```python
from build123d import *

# Parameters (mm, degrees)
SKETCH1_R           = 4
BOSS_EXTRUDE1_DEPTH = 8
CHAMFER1_SIZE       = 0.25
CUT_EXTRUDE1_DEPTH  = 3
CHAMFER2_SIZE       = 0.25


with BuildPart() as part:
    # Sketch1 → Boss-Extrude1 (new body)
    with BuildSketch(Plane(origin=(0, 0, 0), x_dir=(1, 0, 0), z_dir=(0, 1, 0))):
        with Locations(Location((0, 0, 0), (0, 0, 270))):
            Circle(SKETCH1_R)
    extrude(amount=-BOSS_EXTRUDE1_DEPTH)

    # Chamfer1
    chamfer1_edges = [part.edges().sort_by_distance(p)[0] for p in [
        (0, 0, -4),
        (0, -8, -4),
    ]]
    chamfer(chamfer1_edges, length=CHAMFER1_SIZE)

    # Sketch2 → Cut-Extrude1 (cut)
    with BuildSketch(Plane(origin=(0, 0, 0), x_dir=(1, 0, 0), z_dir=(0, 1, 0))):
        Polygon((0, 2.309401077), (2, 1.154700538), (2, -1.154700538), (0, -2.309401077), (-2, -1.154700538), (-2, 1.154700538), align=None)
    extrude(amount=-CUT_EXTRUDE1_DEPTH, mode=Mode.SUBTRACT)

    # Chamfer2
    chamfer2_edges = [part.edges().sort_by_distance(p)[0] for p in [
        (-1, 0, -1.732050808),
        (-2, 0, 0),
        (-1, 0, 1.732050808),
        (1, 0, 1.732050808),
        (2, 0, 0),
        (1, 0, -1.732050808),
    ]]
    chamfer(chamfer2_edges, length=CHAMFER2_SIZE)


solid = part.part
```
Geometry: final body of the model. Coordinates: model frame, mm. A direction names the side the tool comes from. Give positions to 0.01 mm unless a question says otherwise; leave off trailing zeros. Write each loop counter-clockwise with the first axis right and the second up, starting at its lowest first coordinate (ties: lowest second). Pieces come first, ordered by that corner, then holes.
1. Section query C-C, the plane y = -3.5. Return loops of the section in (x, z), then the cut area to 3 significant figures.
2. Section query B-B, the plane z = 0. Return loops of the section in (x, y).
3. Pin query (flat end, axial travel): P1, Ø4, axis at x = -1.5, y = -2, coming from the -Z side; P2, Ø1.5, axis at x = 2.5, y = -3.5, coming from the +Z side; P3, Ø1, axis at y = -5, z = -1, coming from the -X side. Return the tip coordinate at first contact, or that it passes through.
4. Section query A-A, the plane y = -1.5. Return loops of the section in (x, z).
5. Line query: probe 1 along X at (y, z) = (-0.75, -2); probe 2 along Z at (x, y) = (-1.5, -2.5); probe 3 along Z at (x, y) = (3, -2.25). Output: solid intervals per line, ascending.
6. Draft query along Z for faces 1 (the flat face through (1.046, -0.127, -1.848)), 2 (the flat face through (0, -8, 0)), 3 (the cylindrical face through (-3.905, -3.948, -0.867)). Return one class per face: released by +Z, released by -Z, zero draft, split by the parting line, or undercut.
7. Reachability of faces 4 (the flat face through (-2, -2, 0)), 5 (the flat face through (2, 0, 2)) from +Z, -Z, +X, -X, +Y, -Y: full face, straight path, thin tool, end or side. Return the list, or none.
Computed:
1. outline: circle Ø8 at (0, 0)
1. area: 50.3 mm2
2. outline: (-4, -7.75) - (-3.75, -8) - (3.75, -8) - (4, -7.75) - (4, -0.25) - (3.75, 0) - (2.25, 0) - (2, -0.25) - (2, -3) - (-2, -3) - (-2, -0.25) - (-2.25, 0) - (-3.75, 0) - (-4, -0.25) - close
3. P1: stops at z = -4
3. P2: stops at z = 3.6
3. P3: stops at x = -3.97
4. outline: circle Ø8 at (0, 0); hole (-2, -1.15) - (0, -2.31) - (2, -1.15) - (2, 1.15) - (0, 2.31) - (-2, 1.15) - close
5. probe 1: x = -3.46 to -0.54, 0.54 to 3.46
5. probe 2: z = -3.71 to -1.44, 1.44 to 3.71
5. probe 3: z = -2.65 to 2.65
6. face 1: undercut
6. face 2: zero draft
6. face 3: split by the parting line
7. face 4: +Y
7. face 5: +Z, -Z, +X, -X, +Y
